```python
from build123d import *

# Parameters (mm, degrees)
F0_W     = 220
F0_H     = 140
F1_DEPTH = 2
F2_W     = 220
F2_H     = 140
F2_W_2   = 214
F2_H_2   = 134
F3_DEPTH = 30
F4_W     = 217.5
F4_H     = 137.5
F4_W_2   = 214
F4_H_2   = 134
F5_DEPTH = 2


with BuildPart() as f1:
    # F0 (on Top) → F1 (new body)
    with BuildSketch(Plane.XY):
        Rectangle(F0_W, F0_H)
    extrude(amount=F1_DEPTH)

    # F2 (on face) → F3 (join)
    with BuildSketch(Plane.XY.offset(2)):
        Rectangle(F2_W, F2_H)
        Rectangle(F2_W_2, F2_H_2, mode=Mode.SUBTRACT)
    extrude(amount=F3_DEPTH)

    # F4 (on face) → F5 (join)
    with BuildSketch(Plane.XY.offset(32)):
        Rectangle(F4_W, F4_H)
        Rectangle(F4_W_2, F4_H_2, mode=Mode.SUBTRACT)
    extrude(amount=F5_DEPTH)


solid = f1.part
```
Work out the finished part from the listing and answer in its coordinate system (mm). A direction names the side the tool comes from. Round coordinates to 2 decimals unless told otherwise and drop trailing zeros. Write each loop counter-clockwise with the first axis right and the second up, starting at its lowest first coordinate (ties: lowest second). Pieces come first, ordered by that corner, then holes. Notation, with made-up numbers: (-2.5, 51.25) - (14.5, 51.25) arc R21 ccw to (14.5, 56.25) - close; hole circle Ø2 at (24.25, 73.5). An arc over 180 degrees is marked (long way). Return JSON: item names as keys, results as strings. Group by question number.
Q1. The part is cut by section C-C on x = 65.5. Write down the section's boundary in (y, z), then the cut area to 3 significant figures.
Q2. For faces 1 (the flat face through (110, -1, 16)), 2 (the flat face through (107, -1, 18)), determine the directions among +Z, -Z, +X, -X, +Y, -Y from which every point of the face is accessible in a straight line to the end or side of a thin tool.
Q3. The mould has two halves that part along Y. Classify faces 3 (the flat face through (-107, -1, 18)), 4 (the flat face through (-2, 1, 0)), 5 (the flat face through (-2, -70, 16)): released by +Y, released by -Y, zero draft, split by the parting line, or undercut.
Q4. The part is cut by section A-A on z = 15. Write down the section's boundary in (x, y).
Q5. Each of these flat-tipped pins is pushed along its axis until it touches: pin 1 Ø1 at (x, y) = (26.5, 8.5) entering from +Z; pin 2 Ø0.6 at (y, z) = (-9, 33) entering from -X; pin 3 Ø0.6 at (y, z) = (10, 33) entering from +X. Where does it stop, or does it pass through?
Q6. The part is cut by section B-B on y = 61. Write down the section's boundary in (x, z), then the cut area to 3 significant figures.
Q7. Find the intervals of material crossed by L1, parallel to X at y = 38.5, z = 29.5; L2, parallel to Y at x = -80.5, z = 11.5; L3, parallel to Z at x = -62.5, y = -22, in increasing order.
Solved:
{
 "1": {"outline": "(-70, 0) - (70, 0) - (70, 32) - (68.75, 32) - (68.75, 34) - (67, 34) - (67, 2) - (-67, 2) - (-67, 34) - (-68.75, 34) - (-68.75, 32) - (-70, 32) - close", "area": "467 mm²"},
 "2": {"face 1": "+Z, -Z, +X, +Y, -Y", "face 2": "+Z"},
 "3": {"face 3": "undercut", "face 4": "zero draft", "face 5": "released by -Y"},
 "4": {"outline": "(-110, -70) - (110, -70) - (110, 70) - (-110, 70) - close; hole (-107, -67) - (107, -67) - (107, 67) - (-107, 67) - close"},
 "5": {"pin 1": "z = 2", "pin 2": "x = -108.75", "pin 3": "x = 108.75"},
 "6": {"outline": "(-110, 0) - (110, 0) - (110, 32) - (108.75, 32) - (108.75, 34) - (107, 34) - (107, 2) - (-107, 2) - (-107, 34) - (-108.75, 34) - (-108.75, 32) - (-110, 32) - close", "area": "627 mm²"},
 "7": {"L1": "-110 to -107, 107 to 110", "L2": "-70 to -67, 67 to 70", "L3": "0 to 2"}
}
